CAD build for the part. Positions are in the model's coordinates, mm. A direction names the side the tool comes from. Give positions to 0.01 mm unless a question says otherwise; leave off trailing zeros. Write each loop counter-clockwise with the first axis right and the second up, starting at its lowest first coordinate (ties: lowest second). Pieces come first, ordered by that corner, then holes. Notation, with made-up numbers: M 36,61.25 L 92,61.25 A6 cw 92,66.25 Z; hole C -22.5,11 d1. An arc over 180 degrees is marked long. One line per question, with ' | ' between items. Start each with the question number.
1. Pull direction X, two halves, no side cores. Call faces 1 (the face through (20, 5, 2)), 2 (the face through (-18.722, 2.465, 0.216)): released by +X, released by -X, zero draft, split by the parting line, or undercut.
2. Which spindle directions (+Z, -Z, +X, -X, +Y, -Y) get a long thin tool onto all of the face, cutting with end or side? Do faces 3 (the face through (0, 0, 0)), 4 (the face through (-20, 5, 2)), 5 (the face through (0, 10, -12.94)). Say none if no direction does.
3. Cut at A-A, the plane z = 0. Write the cut outline in (x, y), then the cut area to 3 significant figures.
4. Cut at D-D, the plane z = -8.5. Write the cut outline in (x, y).
5. Cut at C-C, the plane x = 5. Write the cut outline in (y, z), then the cut area to 3 significant figures.
6. Cut at B-B, the plane y = 9. Write the cut outline in (x, z).
7. Flat gauge pins, fed straight in: pin 1 (12 mm diameter, centred on x = 7, z = 9.5, fed in from +Y); pin 2 (4 mm diameter, centred on y = 5, z = 9, fed in from +X); pin 3 (4 mm diameter, centred on y = 6.5, z = 4, fed in from +X); pin 4 (5.5 mm diameter, centred on x = -20.37, z = 0, fed in from +Y). Where does each tip first touch, or does it go through?
8. Wall check: L1, parallel to Z at x = 5.5, y = 12; L2, parallel to X at y = 10.5, z = -2.5; L3, parallel to X at y = 5.25, z = 12.5. Give the ranges that are in metal, low to high.
```python
from build123d import *

# Parameters (mm, degrees)
SKETCH1_W           = 35
SKETCH1_H           = 35
BOSS_EXTRUDE1_DEPTH = 13
SKETCH2_W           = 25.47118856
SKETCH2_H           = 25.879985414
CUT_EXTRUDE1_DEPTH  = 7
BOSS_EXTRUDE2_DEPTH = 5
SKETCH5_R           = 1.659140746
CUT_EXTRUDE2_DEPTH  = 33.909124542


with BuildPart() as part:
    # Sketch1 → Boss-Extrude1 (new body)
    with BuildSketch(Plane(origin=(0, 0, 0), x_dir=(1, 0, 0), z_dir=(0, 1, 0))):
        Rectangle(SKETCH1_W, SKETCH1_H)
    extrude(amount=BOSS_EXTRUDE1_DEPTH)

    # Sketch2 → Cut-Extrude1 (cut)
    with BuildSketch(Plane(origin=(0, 13, 0), x_dir=(1, 0, 0), z_dir=(0, 1, 0))):
        Rectangle(SKETCH2_W, SKETCH2_H)
    extrude(amount=-CUT_EXTRUDE1_DEPTH, mode=Mode.SUBTRACT)

    # Sketch3 → Boss-Extrude2 (add)
    with BuildSketch(Plane.XZ):
        with BuildLine():
            Line((-17.5, -5.015622933), (-17.5, 5.83321664))
            ThreePointArc((-17.5, 5.83321664), (-24.652798585, 0.408796853), (-17.5, -5.015622933))
        make_face()
        with BuildLine():
            ThreePointArc((17.5, -5.015622933), (24.652798585, 0.408796853), (17.5, 5.83321664))
            Line((17.5, 5.83321664), (17.5, -5.015622933))
        make_face()
    extrude(amount=-BOSS_EXTRUDE2_DEPTH)

    # Sketch5 → Cut-Extrude2 (cut, through all)
    with BuildSketch(Plane.XZ):
        with Locations(Location((-20.367399271, 0, 0), (0, 0, 270))):
            Circle(SKETCH5_R)
        with Locations(Location((20.367399271, 0, 0), (0, 0, 270))):
            Circle(SKETCH5_R)
    extrude(amount=-CUT_EXTRUDE2_DEPTH, mode=Mode.SUBTRACT)


solid = part.part
```
Here are the results:
1) face 1: zero draft | face 2: undercut
2) face 3: +Z, -Z, +X, -X, -Y | face 4: +Z, -Z, -X, +Y | face 5: +Y
3) outline: M -24.64,0 L -22.03,0 L -22.03,5 L -24.64,5 Z; M -18.71,0 L 18.71,0 L 18.71,5 L 17.5,5 L 17.5,13 L 12.74,13 L 12.74,6 L -12.74,6 L -12.74,13 L -17.5,13 L -17.5,5 L -18.71,5 Z; M 22.03,0 L 24.64,0 L 24.64,5 L 22.03,5 Z | area: 315 mm^2
4) outline: M -17.5,0 L 17.5,0 L 17.5,13 L 12.74,13 L 12.74,6 L -12.74,6 L -12.74,13 L -17.5,13 Z
5) outline: M 0,-17.5 L 13,-17.5 L 13,-12.94 L 6,-12.94 L 6,12.94 L 13,12.94 L 13,17.5 L 0,17.5 Z | area: 274 mm^2
6) outline: M -17.5,-17.5 L 17.5,-17.5 L 17.5,17.5 L -17.5,17.5 Z; hole M -12.74,-12.94 L 12.74,-12.94 L 12.74,12.94 L -12.74,12.94 Z
7) pin 1: y = 13 | pin 2: x = 17.5 | pin 3: x = 24.18 | pin 4: y = 5
8) L1: -17.5 to -12.94, 12.94 to 17.5 | L2: -17.5 to -12.74, 12.74 to 17.5 | L3: -17.5 to 17.5
